from build123d import *

# Parameters (mm, degrees)
SKETCH1_R           = 6
BOSS_EXTRUDE1_DEPTH = 1


with BuildPart() as part:
    # Sketch1 → Boss-Extrude1 (new body)
    with BuildSketch(Plane(origin=(0, 0, 0), x_dir=(1, 0, 0), z_dir=(0, 1, 0))):
        with BuildLine():
            Line((-246.822195025, 82.048831977), (-275.290477825, 91.512281372))
            ThreePointArc((-275.290477825, 91.512281372), (-290.102300616, 0), (-275.290477825, -91.512281372))
            Line((-275.290477825, -91.512281372), (-246.822195025, -82.048831977))
            Line((-246.822195025, -82.048831977), (-237.35874563, -110.517114777))
            Line((-237.35874563, -110.517114777), (-292.692887429, -128.911334562))
            ThreePointArc((-292.692887429, -128.911334562), (-311.881352351, -70.832764917), (-319.66226604, -10.163375435))
            Line((-319.66226604, -10.163375435), (-350.484670263, -10.163375435))
            Line((-350.484670263, -10.163375435), (-350.484670263, 10.163375435))
            Line((-350.484670263, 10.163375435), (-319.66226604, 10.163375435))
            ThreePointArc((-319.66226604, 10.163375435), (-311.881352351, 70.832764917), (-292.692887429, 128.911334562))
            Line((-292.692887429, 128.911334562), (-237.35874563, 110.517114777))
            Line((-237.35874563, 110.517114777), (-246.822195025, 82.048831977))
        make_face()
        with Locations(Location((-332.928005197, 0, 0), (0, 0, 270))):
            Circle(SKETCH1_R, mode=Mode.SUBTRACT)
    extrude(amount=BOSS_EXTRUDE1_DEPTH)


solid = part.part
Verification items for the finished model (mm, model axes). A direction names the side the tool comes from. Give positions to 0.01 mm unless a question says otherwise; leave off trailing zeros. Order: outer loops, then holes, each group sorted by start corner. A loop starts at its lowest first (then second) coordinate and runs counter-clockwise, first axis right, second up. Notation, with made-up numbers: M 78.25,31 L 91.25,31 A20 ccw 91.25,59 Z; hole C -25,-15.5 d11. An arc over 180 degrees is marked long. Use one line per item in the form item = value. Start each with the question number.
Q1. Access from +Z, -Z, +X, -X, +Y, -Y to the whole of each face (thin tool, end or side, straight path). Record for faces 4 (the flat face through (-261.26, 0.49, 86.85)), 5 (the flat face through (-242.16, 0.49, 96.08)), 6 (the flat face through (-294, 0, 9)).
Q2. Section check B-B (x = -257). Enter the section's corners in (y, z).
Q3. Section check C-C (y = 0.45). Enter the section's corners in (x, z), then the cut area to 3 significant figures.
Q4. Mould release check, pull along X, two halves, no side actions. Record for faces 1 (the cylindrical face through (-338.25, 0.49, 2.77)), 2 (the flat face through (-264.638, 0.493, 119.585)), 3 (the flat face through (-294, 1, 9)): +X half, -X half, draft (parallel to the pull), parting line (faces both ways), or undercut.
Q5. Section check A-A (z = 0). Enter the section's corners in (x, y), then the cut area to 3 significant figures.
Q6. Scan lines: line 1 along X through (y, z) = (0.4, 0); line 2 along Z through (x, y) = (-341, 0.2); line 3 along Z through (x, y) = (-329.5, 0.2). Record each from-to range of solid material in increasing order. Write a range as [from, to].
Q7. Section check D-D (x = -322). Enter the section's corners in (y, z), then the cut area to 3 significant figures.
Evaluation:
q1.face_4 = +Y, -Y
q1.face_5 = +X, +Y, -Y
q1.face_6 = +Z, -Z, +X, -X, -Y
q2.outline = M 0,-117.05 L 1,-117.05 L 1,-85.43 L 0,-85.43 Z; M 0,85.43 L 1,85.43 L 1,117.05 L 0,117.05 Z
q3.outline = M -350.48,-10.16 L -319.66,-10.16 A319.82 ccw -292.69,-128.91 L -237.36,-110.52 L -246.82,-82.05 L -275.29,-91.51 A290.1 cw -275.29,91.51 L -246.82,82.05 L -237.36,110.52 L -292.69,128.91 A319.82 ccw -319.66,10.16 L -350.48,10.16 Z; hole C -332.93,0 d12
q3.area = 9,880 mm2
q4.face_1 = undercut
q4.face_2 = +X half
q4.face_3 = draft
q5.outline = M -350.48,0 L -338.93,0 L -338.93,1 L -350.48,1 Z; M -326.93,0 L -290.1,0 L -290.1,1 L -326.93,1 Z
q5.area = 48.4 mm2
q6.line_1 = [-350.48, -338.93], [-326.93, -290.1]
q6.line_2 = [-10.16, 10.16]
q6.line_3 = [-10.16, -4.92], [4.92, 10.16]
q7.outline = M 0,-10.16 L 1,-10.16 L 1,10.16 L 0,10.16 Z
q7.area = 20.3 mm2
